```python
from build123d import *

# Parameters (mm, degrees)
BOSS_EXTRUDE1_DEPTH   = 25
BOSS_EXTRUDE1_2_DEPTH = 25
BOSS_EXTRUDE2_DEPTH   = 2
SKETCH2_W             = 18.3
SKETCH2_H             = 6.5
BOSS_EXTRUDE3_DEPTH   = 6.5
CUT_EXTRUDE1_REACH    = 46.322
SKETCH3_R             = 1.45
CUT_EXTRUDE3_REACH    = 40.862
SKETCH4_R             = 1.7


with BuildPart() as part:
    # Sketch1 → Boss-Extrude1 (new body)
    with BuildSketch(Plane(origin=(0, 0, 0), x_dir=(1, 0, 0), z_dir=(0, 1, 0))):
        Polygon((-11, -25.5), (-15, -25.5), (-15, -27.5), (15, -27.5), (15, -25.5), (11, -25.5), (11, -26), (9.15, -26), (9.15, -25.5), (-9.15, -25.5), (-9.15, -26), (-11, -26), align=None)
    extrude(amount=BOSS_EXTRUDE1_DEPTH)



with BuildPart() as body_2:
    # Sketch1 → Boss-Extrude1 2 (new body)
    with BuildSketch(Plane(origin=(0, 0, 0), x_dir=(1, 0, 0), z_dir=(0, 1, 0))):
        Polygon((15, 27.5), (-15, 27.5), (-15, 25.5), (-11, 25.5), (-11, 26), (-9.15, 26), (-9.15, 25.5), (9.15, 25.5), (9.15, 26), (11, 26), (11, 25.5), (15, 25.5), align=None)
    extrude(amount=BOSS_EXTRUDE1_2_DEPTH)


with BuildPart() as part_1:
    add(part.part)

    add(body_2.part)  # Boss-Extrude2 merges body 2
    # Sketch1_3 → Boss-Extrude2 (add)
    with BuildSketch(Plane(origin=(0, 0, 0), x_dir=(1, 0, 0), z_dir=(0, 1, 0))):
        Polygon((-11, 25.5), (-15, 25.5), (-15, -25.5), (-11, -25.5), (-11, -26), (-9.15, -26), (-9.15, -25.5), (9.15, -25.5), (9.15, -26), (11, -26), (11, -25.5), (15, -25.5), (15, 25.5), (11, 25.5), (11, 26), (9.15, 26), (9.15, 25.5), (-9.15, 25.5), (-9.15, 26), (-11, 26), align=None)
    extrude(amount=BOSS_EXTRUDE2_DEPTH)

    # Sketch2 → Boss-Extrude3 (add)
    with BuildSketch(Plane(origin=(0, 2, 0), x_dir=(1, 0, 0), z_dir=(0, 1, 0))):
        with Locations((0, -22.25)):
            Rectangle(SKETCH2_W, SKETCH2_H)
    boss_extrude3 = extrude(amount=BOSS_EXTRUDE3_DEPTH)

    # Sketch3 → Cut-Extrude1 (cut, up to next)
    with BuildSketch(Plane(origin=(9.15, 0, 0), x_dir=(0, 0, -1), z_dir=(1, 0, 0)), mode=Mode.PRIVATE) as cut_extrude1_sk1:
        with Locations((-21.7, 5.8)):
            Circle(SKETCH3_R)
    cut_extrude1_tool1 = extrude(cut_extrude1_sk1.sketch, amount=-CUT_EXTRUDE1_REACH, mode=Mode.PRIVATE) & part_1.part
    cut_extrude1 = cut_extrude1_tool1.solids().sort_by_distance((9.15, 5.8, 21.7))[0]
    add(cut_extrude1, mode=Mode.SUBTRACT)

    # Sketch4 → Cut-Extrude3 (cut, up to next)
    with BuildSketch(Plane(origin=(0, 2, 0), x_dir=(1, 0, 0), z_dir=(0, 1, 0)), mode=Mode.PRIVATE) as cut_extrude3_sk1:
        with Locations(Location((0, 10, 0), (0, 0, 270))):
            Circle(SKETCH4_R)
    cut_extrude3_tool1 = extrude(cut_extrude3_sk1.sketch, amount=-CUT_EXTRUDE3_REACH, mode=Mode.PRIVATE) & part_1.part
    # Sketch4 → Cut-Extrude3 (cut, up to next)
    with BuildSketch(Plane(origin=(0, 2, 0), x_dir=(1, 0, 0), z_dir=(0, 1, 0)), mode=Mode.PRIVATE) as cut_extrude3_sk2:
        with Locations(Location((0, -10, 0), (0, 0, 270))):
            Circle(SKETCH4_R)
    cut_extrude3_tool2 = extrude(cut_extrude3_sk2.sketch, amount=-CUT_EXTRUDE3_REACH, mode=Mode.PRIVATE) & part_1.part
    add(cut_extrude3_tool1.solids().sort_by_distance((0, 2, -10))[0], mode=Mode.SUBTRACT)
    add(cut_extrude3_tool2.solids().sort_by_distance((0, 2, 10))[0], mode=Mode.SUBTRACT)

    # Mirror1: Boss-Extrude3, Cut-Extrude1 across plane
    add(boss_extrude3.mirror(Plane.XY))
    add(cut_extrude1.mirror(Plane.XY), mode=Mode.SUBTRACT)


solid = part_1.part
```
Design review of the part built by this model. Coordinates are the model's own, in mm. A direction names the side the tool comes from. Give positions to 0.01 mm unless a question says otherwise; leave off trailing zeros. Write each loop counter-clockwise with the first axis right and the second up, starting at its lowest first coordinate (ties: lowest second). Pieces come first, ordered by that corner, then holes. Notation, with made-up numbers: (79, 23) - (115, 23) arc R23 cw to (115, 43) - close; hole circle Ø11 at (88.5, 33.25). An arc over 180 degrees is marked (long way). Return JSON: item names as keys, results as strings. Group by question number.
(1) Machinability: for faces 4 (the flat face through (9.15, 8, -23)), 5 (the flat face through (-13, 13, 25.5)), 6 (the flat face through (0, 5, 19)), which of the approach directions +Z, -Z, +X, -X, +Y, -Y give a long, thin tool a straight path to every point of the face, cutting with its end or side? Answer none if there is none.
(2) We need section D-D, the plane x = 7.75. Give the boundary of the cut face in (y, z), then the cut area to 3 significant figures.
(3) We need section C-C, the plane z = -21.7. Give the boundary of the cut face in (x, y), then the cut area to 3 significant figures.
(4) Insertion check: pin 1 (7 mm diameter, centred on x = -1, z = 23.5, fed in from +Y); pin 2 (7.5 mm diameter, centred on y = 10, z = -21.5, fed in from +X); pin 3 (5 mm diameter, centred on x = -4, z = -21, fed in from +Y); pin 4 (4.5 mm diameter, centred on y = 5.8, z = -21.7, fed in from -X). Each pin has a flat end and moves straight along its axis. Give the tip position at first contact, or say it passes through.
(5) To check wall thickness, follow probe 1 along X at (y, z) = (1.4, 10); probe 2 along Y at (x, z) = (-3, 21.7); probe 3 along Z at (x, y) = (1, 6.5). State the ranges of each line that lie inside material, in increasing order.
(6) We need section A-A, the plane x = 0. Give the boundary of the cut face in (y, z).
(7) We need section B-B, the plane y = 11. Give the boundary of the cut face in (x, z), then the cut area to 3 significant figures.
(8) Mouldability with a two-part tool opening along Y and no side actions: class faces 1 (the flat face through (0, 8.5, -22)), 2 (the flat face through (15, 1, 2)), 3 (the cylindrical face through (0.13, 6.78, -22.77)) as +Y half, -Y half, draft (parallel to the pull), parting line (faces both ways), or undercut.
Reported:
{
 "1": {"face 4": "+Y", "face 5": "-X, +Y", "face 6": "+X, -X, +Y"},
 "2": {"outline": "(0, -27.5) - (25, -27.5) - (25, -25.5) - (8.5, -25.5) - (8.5, -19) - (2, -19) - (2, 19) - (8.5, 19) - (8.5, 25.5) - (25, 25.5) - (25, 27.5) - (0, 27.5) - close; hole circle Ø2.9 at (5.8, -21.7); hole circle Ø2.9 at (5.8, 21.7)", "area": "273 mm2"},
 "3": {"outline": "(-15, 0) - (15, 0) - (15, 2) - (9.15, 2) - (9.15, 4.35) - (-9.15, 4.35) - (-9.15, 2) - (-15, 2) - close; (-9.15, 7.25) - (9.15, 7.25) - (9.15, 8.5) - (-9.15, 8.5) - close", "area": "126 mm2"},
 "4": {"pin 1": "stops at y = 25", "pin 2": "stops at x = 9.15", "pin 3": "stops at y = 8.5", "pin 4": "stops at x = -9.15"},
 "5": {"probe 1": "x = -15 to -1.7, 1.7 to 15", "probe 2": "y = 0 to 4.35, 7.25 to 8.5", "probe 3": "z = -27.5 to -22.97, -20.43 to -19, 19 to 20.43, 22.97 to 27.5"},
 "6": {"outline": "(0, -27.5) - (25, -27.5) - (25, -25.5) - (8.5, -25.5) - (8.5, -19) - (2, -19) - (2, -11.7) - (0, -11.7) - close; (0, -8.3) - (2, -8.3) - (2, 8.3) - (0, 8.3) - close; (0, 11.7) - (2, 11.7) - (2, 19) - (8.5, 19) - (8.5, 25.5) - (25, 25.5) - (25, 27.5) - (0, 27.5) - close; hole circle Ø2.9 at (5.8, -21.7); hole circle Ø2.9 at (5.8, 21.7)"},
 "7": {"outline": "(-15, -27.5) - (15, -27.5) - (15, -25.5) - (11, -25.5) - (11, -26) - (9.15, -26) - (9.15, -25.5) - (-9.15, -25.5) - (-9.15, -26) - (-11, -26) - (-11, -25.5) - (-15, -25.5) - close; (-15, 25.5) - (-11, 25.5) - (-11, 26) - (-9.15, 26) - (-9.15, 25.5) - (9.15, 25.5) - (9.15, 26) - (11, 26) - (11, 25.5) - (15, 25.5) - (15, 27.5) - (-15, 27.5) - close", "area": "116 mm2"},
 "8": {"face 1": "+Y half", "face 2": "draft", "face 3": "undercut"}
}
